Autodesk Inventor part; units mm, degrees
ref_plane "YZ Plane" through (0, 0, 0) normal (1, 0, 0) x (0, 1, 0)
ref_plane "XZ Plane" through (0, 0, 0) normal (0, 1, 0) x (-1, 0, 0)
ref_plane "XY Plane" through (0, 0, 0) normal (0, 0, 1) x (1, 0, 0)
sketch "Sketch1" plane through (0, 0, 0) normal (0, 1, 0) x (-1, 0, 0)
  line L0 (20.25, -10) -> (-20.25, -10)
  line L1 (-20.25, -10) -> (-20.25, 10)
  line L2 (-20.25, 10) -> (20.25, 10)
  line L3 (20.25, 10) -> (20.25, -10)
  point P0 (0, 0)
  dimension "d0" = 40.5
  dimension "d1" = 20
  dimension "d2" = 10
  dimension "d3" = 20.25
extrude "Plate1" add sketch "Sketch1" along normal blind 1.5
sketch "Sketch2" plane through (21.75, 0, -10) normal (-1, 0, 0) x (0, -1, 0)
  line L0 (0, 20) -> (0, 0)
  line L1 (0, 0) -> (-43.5, 0)
  line L2 (-43.5, 0) -> (-43.5, 20)
  line L3 (-43.5, 20) -> (0, 20)
edge flange "Flange1" height 43.5 angle 90 thickness 1.5 bend radius 0.31 thickness toward (-1, 0, 0) relief tear relief width 1.5 relief depth 0.75 edges at (20.25, 1.5, 0) wall of the first edge with corners at (21.75, 0, 10) (21.75, 0, -10) (21.75, 43.5, -10) (21.75, 43.5, 10)
bend "Bend1"
corner "Corner1"
sketch "Sketch3" plane through (-21.75, 0, 10) normal (1, 0, 0) x (0, 1, 0)
  line L0 (0, -20) -> (0, 0)
  line L1 (0, 0) -> (43.5, 0)
  line L2 (43.5, 0) -> (43.5, -20)
  line L3 (43.5, -20) -> (0, -20)
edge flange "Flange2" height 43.5 angle 90 thickness 1.5 bend radius 0.31 thickness toward (1, 0, 0) relief tear relief width 1.5 relief depth 0.75 edges at (-20.25, 1.5, 0) wall of the first edge with corners at (-21.75, 0, -10) (-21.75, 0, 10) (-21.75, 43.5, 10) (-21.75, 43.5, -10)
bend "Bend2"
corner "Corner2"
sketch "Sketch4" plane through (21.75, 43.5, 10) normal (1, 0, 0) x (0, 0, -1)
  circle A0 centre (10, -9.9) radius 6.75
  line L0 (0, 0) -> (20, 0)
  line L1 (20, 0) -> (20, -41.69)
  point P0 (10, -43.5)
  dimension "d25" = 9.9
  dimension "d26" = 13.5
  dimension "d27" = 10
extrude "Extrusion1" cut sketch "Sketch4" against normal blind 50
sketch "Sketch5" plane through (21.75, 43.5, 10) normal (1, 0, 0) x (0, 0, -1)
  circle A0 centre (10, -9.9) radius 6.75
  line L0 (0, 0) -> (20, 0)
  line L1 (-4, 0) -> (24, 0)
  line L2 (24, 0) -> (24, -9.9)
  line L3 (24, -9.9) -> (-4, -9.9)
  line L4 (-4, -9.9) -> (-4, 0)
  line L5 (0, -41.69) -> (0, 0)
  point P0 (10, -43.5)
  point P1 (20, 0)
  dimension "d30" = 9.9
  dimension "d31" = 28
  dimension "d32" = 4
extrude "Extrusion2" cut sketch "Sketch5" against normal blind 50 contours L3 A0 | A0 L3 L5 L0 L1 L2 | L3 L4 L1 L5 picked at (11.6841, -8.408)
fillet "Fillet1" radius 1 4 edges at (-21, 33.6, 10) (-21, 33.6, -10) (21, 33.6, -10) (21, 33.6, 10)
sketch "Sketch11" plane through (0, 1.5, 0) normal (0, 1, 0) x (1, 0, 0)
  circle A0 centre (7, 7) radius 1.5
  line L0 (-19.94, 10) -> (19.94, 10)
  line L1 (-19.94, 10) -> (-19.94, -10)
  circle A1 centre (-7, 7) radius 1.5
  circle A2 centre (7, -7) radius 1.5
  circle A3 centre (-7, -7) radius 1.5
  point P0 (0, 0)
  dimension "d71" = 7
  dimension "d72" = 3
  dimension "d73" = 7
  dimension "d76" = 14
  dimension "d79" = 14
extrude "Extrusion3" cut sketch "Sketch11" against normal through all
sketch "Sketch12" plane through (-21.75, 1.81, -10) normal (-1, 0, 0) x (0, 0, 1)
  circle A0 centre (18, 24.89) radius 0.7835
  circle A1 centre (10, 24.79) radius 0.7835
  circle A2 centre (17, 11.67) radius 0.7835
  circle A3 centre (3, 11.67) radius 0.7835
  circle A4 centre (10, 4.37) radius 0.7835
  circle A5 centre (2, 24.89) radius 0.7835
  point P0 (10, -1.81)
hole "Hole6" at (-21.75, 26.7, -8) at (-21.75, 26.7, 8) at (-21.75, 13.48, 7) at (-21.75, 6.18, 0) at (-21.75, 13.48, -7) direction (1, 0, 0) diameter 2.1 depth 1.5
sketch "Sketch13" plane through (21.75, 1.81, 10) normal (1, 0, 0) x (0, 0, -1)
  circle A0 centre (17.525, 4.19) radius 0.7835
  circle A1 centre (2.475, 4.19) radius 0.7835
  circle A2 centre (2.475, 19.29) radius 0.7835
  circle A3 centre (17.525, 19.29) radius 0.7835
  point P0 (10, -1.81)
hole "Hole7" at (21.75, 21.1, 7.525) at (21.75, 21.1, -7.525) at (21.75, 6, -7.525) at (21.75, 6, 7.525) direction (-1, 0, 0) diameter 2.1 depth 1.5
equation "\"d89\" = Thickness"
equation "\"d96\" = Thickness"
equation "\"d4\" = Thickness"
equation "\"d5\" = BendReliefWidth"
equation "\"d6\" = BendReliefDepth"
equation "\"d7\" = MinimumRemnant"
equation "\"d8\" = TransitionRadius"
equation "\"d11\" = BendRadius"
equation "\"d12\" = CornerReliefSize"
equation "\"d13\" = GapSize"
equation "\"d14\" = JacobiRadiusSize"
equation "\"d15\" = BendReliefWidth"
equation "\"d16\" = BendReliefDepth"
equation "\"d17\" = MinimumRemnant"
equation "\"d18\" = TransitionRadius"
equation "\"d21\" = BendRadius"
equation "\"d22\" = CornerReliefSize"
equation "\"d23\" = GapSize"
equation "\"d24\" = JacobiRadiusSize"
equation "\"BendReliefWidth\" = Thickness"
equation "\"BendReliefDepth\" = 0.5 * Thickness"
equation "\"CornerReliefSize\" = 4 * Thickness"
equation "\"MinimumRemnant\" = 2 * Thickness"
equation "\"TransitionRadius\" = BendRadius"
equation "\"JacobiRadiusSize\" = BendRadius"
equation "\"GapSize\" = Thickness"
properties part number "axis_10_top_frame" material "Aluminum 6061-AHC"
Model file for the job. Use its own axes, mm. A direction names the side the tool comes from. Give positions to 0.01 mm unless a question says otherwise; leave off trailing zeros. Loops run counter-clockwise (first coordinate to the right, second up) from the corner with the lowest first, then second, coordinate; pieces in that order, holes last.
1) Tool access for faces 1 (the flat face through (0, 1.5, 0)), 2 (the flat face through (21, 33.6, 8)), 3 (the cylindrical face through (20.99, 20.06, 7.66)): list every direction of +Z, -Z, +X, -X, +Y, -Y with a clear straight run to the whole face (end or side of a thin tool).
2) Saw through at C-C (y = 29). Write the cut outline in (x, z).
3) Saw through at A-A (y = 21.1). Write the cut outline in (x, z) (3 decimals).
4) Flat gauge pins, fed straight in: pin 1 Ø6 at (x, z) = (1, 3) entering from +Y; pin 2 Ø1.7 at (y, z) = (13.48, -7) entering from -X. Where does each tip first touch, or does it go through?
5) Wall check: line 1 (Z direction, x = -7, y = 0.75); line 2 (Z direction, x = -20.7, y = 13.48); line 3 (X direction, y = 3, z = -3). Give the ranges that are in metal, low to high.
6) Pull direction Y, two halves, no side cores. Call faces 4 (the cylindrical face through (-20.99, 27.725, -8.228)), 5 (the cylindrical face through (20.99, 33.299, 9.715)), 6 (the flat face through (-20.25, 17, 0)), 7 (the cylindrical face through (-20.99, 7.205, -0.228)): +Y half, -Y half, draft (parallel to the pull), parting line (faces both ways), or undercut.
7) Saw through at B-B (x = 4.5). Write the cut outline in (y, z).
Answer block:
1. face 1: +Z, -Z, +Y
1. face 2: +Z, -Z, +X, -X, +Y
1. face 3: +X
2. outline: (-21.75, -10) - (-20.25, -10) - (-20.25, -4.94) - (-21.75, -4.94) - close; (-21.75, 4.94) - (-20.25, 4.94) - (-20.25, 10) - (-21.75, 10) - close; (20.25, -10) - (21.75, -10) - (21.75, -4.94) - (20.25, -4.94) - close; (20.25, 4.94) - (21.75, 4.94) - (21.75, 10) - (20.25, 10) - close
3. outline: (-21.75, -10) - (-20.25, -10) - (-20.25, 10) - (-21.75, 10) - close; (20.25, -10) - (21.75, -10) - (21.75, -8.575) - (20.25, -8.575) - close; (20.25, -6.475) - (21.75, -6.475) - (21.75, 6.475) - (20.25, 6.475) - close; (20.25, 8.575) - (21.75, 8.575) - (21.75, 10) - (20.25, 10) - close
4. pin 1: stops at y = 1.5
4. pin 2: stops at x = 20.25
5. line 1: z = -10 to -8.5, -5.5 to 5.5, 8.5 to 10
5. line 2: z = -10 to -8.05, -5.95 to 5.95, 8.05 to 10
5. line 3: x = -21.75 to -20.25, 20.25 to 21.75
6. face 4: undercut
6. face 5: +Y half
6. face 6: draft
6. face 7: undercut
7. outline: (0, -10) - (1.5, -10) - (1.5, 10) - (0, 10) - close
